Build history of the part. All positions in model axes, mm. A direction names the side the tool comes from. Round coordinates to 2 decimals unless told otherwise and drop trailing zeros. Write each loop counter-clockwise with the first axis right and the second up, starting at its lowest first coordinate (ties: lowest second). Pieces come first, ordered by that corner, then holes. Notation, with made-up numbers: (0, -10) - (20, -10) arc R12 ccw to (20, 13) - close; hole circle Ø3 at (-25, 75). An arc over 180 degrees is marked (long way). Write each question's results on one line, items separated by ' | '.
from build123d import *

# Parameters (mm, degrees)
SKETCH2_W           = 120
SKETCH2_H           = 250
BOSS_EXTRUDE1_DEPTH = 100
SKETCH4_R           = 20
CUT_EXTRUDE1_DEPTH  = 100
SKETCH5_R           = 20
CUT_EXTRUDE5_DEPTH  = 201.062490237
SCALE1_SCALE        = 0.35


with BuildPart() as part:
    # Sketch2 → Boss-Extrude1 (new body)
    with BuildSketch(Plane(origin=(0, 0, 0), x_dir=(1, 0, 0), z_dir=(0, 1, 0))):
        Rectangle(SKETCH2_W, SKETCH2_H)
    extrude(amount=BOSS_EXTRUDE1_DEPTH)

    # Sketch4 → Cut-Extrude1 (cut)
    with BuildSketch(Plane(origin=(0, 100, 0), x_dir=(1, 0, 0), z_dir=(0, 1, 0))):
        with BuildLine():
            Line((-60, 125), (-60, -17.644609552))
            ThreePointArc((-60, -17.644609552), (-52.622366518, 11.180492718), (-32.303782241, 32.916893747))
            ThreePointArc((-32.303782241, 32.916893747), (-25.530920786, 40.16236081), (-23.071709655, 49.770728302))
            Line((-23.071709655, 49.770728302), (-23.071709655, 125))
            Line((-23.071709655, 125), (-60, 125))
        make_face()
        with BuildLine():
            ThreePointArc((32.303782241, 32.916893747), (52.62236667, 11.18049244), (60, -17.644610185))
            Line((60, -17.644610185), (60, 125))
            Line((60, 125), (23.071709655, 125))
            Line((23.071709655, 125), (23.071709655, 49.770728302))
            ThreePointArc((23.071709655, 49.770728302), (25.530920786, 40.16236081), (32.303782241, 32.916893747))
        make_face()
        with Locations((0, -17.644609919)):
            Circle(SKETCH4_R)
        with BuildLine():
            Line((-20, -17.644609919), (-20, -74.213152414))
            ThreePointArc((-20, -74.213152414), (0, -77.644609919), (20, -74.213152414))
            Line((20, -74.213152414), (20, -17.644609919))
            ThreePointArc((20, -17.644609919), (0, -37.644609919), (-20, -17.644609919))
        make_face()
        with BuildLine():
            Line((-20, -74.213152414), (-20, -125))
            Line((-20, -125), (20, -125))
            Line((20, -125), (20, -74.213152414))
            ThreePointArc((20, -74.213152414), (0, -77.644609919), (-20, -74.213152414))
        make_face()
    extrude(amount=-CUT_EXTRUDE1_DEPTH, mode=Mode.SUBTRACT)

    # Sketch5 → Cut-Extrude5 (cut, through all)
    # profile 1 of 2: a face of its own
    with BuildSketch(Plane(origin=(60, 0, 0), x_dir=(0, 0, -1), z_dir=(1, 0, 0))):
        Polygon((125, 100), (49.770728302, 100), (32.916893747, 100), (-17.644609919, 100), (-125, 100), (-125, 0), (-17.644609919, 0), (32.916893747, 0), (49.770728302, 0), (125, 0), align=None)
        with BuildLine():
            Line((125, 73.474979738), (125, 26.525020262))
            Line((125, 26.525020262), (-20.137206262, 26.525020262))
            ThreePointArc((-20.137206262, 26.525020262), (-28.84270867, 24.530970051), (-35.812290187, 18.946443044))
            ThreePointArc((-35.812290187, 18.946443044), (-125, 50), (-35.812290187, 81.053556956))
            ThreePointArc((-35.812290187, 81.053556956), (-28.84270867, 75.469029949), (-20.137206262, 73.474979738))
            Line((-20.137206262, 73.474979738), (125, 73.474979738))
        make_face(mode=Mode.SUBTRACT)
    # profile 2 of 2: a face of its own
    with BuildSketch(Plane(origin=(60, 0, 0), x_dir=(0, 0, -1), z_dir=(1, 0, 0))):
        with Locations((-75, 50)):
            Circle(SKETCH5_R)
    extrude(amount=-CUT_EXTRUDE5_DEPTH, mode=Mode.SUBTRACT)


with BuildPart() as cut_extrude5_kept_piece:
    # of the separate pieces the step leaves, the one the design keeps (cut_extrude5_pieces_kept)
    add(part.part.solids().sort_by_distance((23.071709655, 73.474979738, -125))[0])


with BuildPart() as cut_extrude5_kept_piece_1:
    # Scale1: scaled about (0, 50, 23.23209908)
    add(cut_extrude5_kept_piece.part.scale(SCALE1_SCALE).moved(Location((0, 32.5, 15.100864402))))


solid = cut_extrude5_kept_piece_1.part
(1) Slice it at A-A, the plane y = 50. Write the cut outline in (x, z).
Worked answers:
outline: (-21, 21.28) arc R21 ccw to (-11.31, 3.58) arc R7 cw to (-8.08, -2.32) - (-8.08, -28.65) - (8.08, -28.65) - (8.08, -2.32) arc R7 cw to (11.31, 3.58) arc R21 ccw to (21, 21.28) - (21, 34.35) - (7, 34.35) - (7, 21.28) arc R7 cw to (-7, 21.28) - (-7, 34.35) - (-21, 34.35) - close; (-21, 48.35) - (-7, 48.35) - (-7, 58.85) - (-21, 58.85) - close; (7, 48.35) - (21, 48.35) - (21, 58.85) - (7, 58.85) - close
(2) Two-plate mould, pull along X, no slides. Class faces 1 (the cylindrical face through (-13.9, 54.73, 46.51)), 2 (the cylindrical face through (18.347, 50.115, 11.059)), 3 (the flat face through (-7, 58, 40)), 4 (the flat face through (-21, 58, 40)): released by +X, released by -X, zero draft, split by the parting line, or undercut.
Worked answers:
face 1: zero draft | face 2: released by +X | face 3: undercut | face 4: released by -X
(3) Drill centre lines: probe 1 along X at (y, z) = (49, 55); probe 2 along X at (y, z) = (42, -11.5); probe 3 along Z at (x, y) = (12, 46). Where is each one in solid material? Low to high. Write a range as [from, to].
Worked answers:
probe 1: x = [-21, -7], [7, 21] | probe 2: x = [-8.08, 8.08] | probe 3: z = [4.04, 35.61], [47.1, 58.39]
(4) Slice it at D-D, the plane y = 44. Write the cut outline in (x, z).
Worked answers:
outline: (-21, 21.28) arc R21 ccw to (-11.31, 3.58) arc R7 cw to (-8.08, -2.32) - (-8.08, -28.65) - (8.08, -28.65) - (8.08, -2.32) arc R7 cw to (11.31, 3.58) arc R21 ccw to (21, 21.28) - (21, 37.75) - (7, 37.75) - (7, 21.28) arc R7 cw to (-7, 21.28) - (-7, 37.75) - (-21, 37.75) - close; (-21, 44.96) - (-7, 44.96) - (-7, 57.79) - (-21, 57.79) - close; (7, 44.96) - (21, 44.96) - (21, 57.79) - (7, 57.79) - close
(5) Flat gauge pins, fed straight in: pin 1 Ø2 at (x, y) = (11.5, 59) entering from -Z; pin 2 Ø5 at (y, z) = (49, -22) entering from +X; pin 3 Ø21 at (x, z) = (6, 0.5) entering from +Y. Where does each tip first touch, or does it go through?
Worked answers:
pin 1: stops at z = 3.28 | pin 2: stops at x = 8.08 | pin 3: stops at y = 58.22
(6) Slice it at B-B, the plane x = 13.5. Write the cut outline in (y, z).
Worked answers:
outline: (39.13, 27.64) arc R7 cw to (41.78, 22.15) - (41.78, 5.19) - (58.22, 5.19) - (58.22, 22.15) arc R7 cw to (60.87, 27.64) arc R17.5 ccw (long way) to start; hole circle Ø14 at (50, 41.35)
(7) Tool access for faces 5 (the flat face through (0, 58.216, 3)), 6 (the flat face through (8.075, 50, -16)), 7 (the flat face through (-8.075, 50, -15)), 8 (the flat face through (0, 41.784, 2)), 9 (the cylindrical face through (14.1, 49.39, 58.84)): list every direction of +Z, -Z, +X, -X, +Y, -Y with a clear straight run to the whole face (end or side of a thin tool).
Worked answers:
face 5: -Z, +X, -X, +Y | face 6: -Z, +X, +Y, -Y | face 7: -Z, -X, +Y, -Y | face 8: -Z, +X, -X, -Y | face 9: +X, -X
(8) Slice it at C-C, the plane z = 52. Write the cut outline in (x, y).
Worked answers:
outline: (-21, 36.11) - (-7, 36.11) - (-7, 63.89) - (-21, 63.89) - close; (7, 36.11) - (21, 36.11) - (21, 63.89) - (7, 63.89) - close
